Input: part model. Units: mm. Frame: model coordinates. A direction names the side the tool comes from. Round coordinates to 2 decimals unless told otherwise and drop trailing zeros. Order: outer loops, then holes, each group sorted by start corner. A loop starts at its lowest first (then second) coordinate and runs counter-clockwise, first axis right, second up.
Item 1: Cut plane D-D on y = -0.5. Output: boundary loops of the cut face in (x, z).
Item 2: Reachability of faces 1 (the flat face through (0, -33, 0)), 2 (the cylindrical face through (32.809, -3.2, 45.205)), 3 (the flat face through (-26.212, -3, 173)) from +Z, -Z, +X, -X, +Y, -Y: full face, straight path, thin tool, end or side. Return the list, or none.
Item 3: Line query: L1, parallel to X at y = 9, z = 141; L2, parallel to Y at x = 11.5, z = 141. Output: solid intervals per line, ascending.
Item 4: Cut plane C-C on z = 114.5. Output: boundary loops of the cut face in (x, y).
Item 5: Mould query, pull axis Y, two halves, no side actions, for faces 4 (the flat face through (-29.212, -3, 173)), 5 (the flat face through (2, -34.267, 173)), 6 (the flat face through (2, 29.233, 173)), 7 (the flat face through (2, 26.233, 173)). Classes: released by +Y, released by -Y, zero draft, split by the parting line, or undercut.
Item 6: Cut plane A-A on x = -7. Output: boundary loops of the cut face in (y, z), then the cut area to 3 significant figures.
Item 7: Cut plane B-B on y = 15.5. Output: boundary loops of the cut face in (x, z).
```python
from build123d import *

# Parameters (mm, degrees)
F0_W     = 63.5
F0_H     = 63.5
F0_W_2   = 57.5
F0_H_2   = 57.5
F1_DEPTH = 350
F2_R     = 5.25
F3_DEPTH = 10


with BuildPart() as f1:
    # F0 (on Top) → F1 (new body)
    with BuildSketch(Plane.XY):
        with Locations((2.538389, -2.516717)):
            Rectangle(F0_W, F0_H)
        with Locations((2.538389, -2.516717)):
            Rectangle(F0_W_2, F0_H_2, mode=Mode.SUBTRACT)
    extrude(amount=F1_DEPTH)

    # F2 (on face) → F3 (cut)
    with BuildSketch(Plane.YZ.offset(34.288389)):
        with Locations((-2.516717, 40)):
            Circle(F2_R)
    extrude(amount=-F3_DEPTH, mode=Mode.SUBTRACT)


solid = f1.part
```
From the geometry:
1. outline: (-29.21, 0) - (-26.21, 0) - (-26.21, 350) - (-29.21, 350) - close; (31.29, 0) - (34.29, 0) - (34.29, 35.15) - (31.29, 35.15) - close; (31.29, 44.85) - (34.29, 44.85) - (34.29, 350) - (31.29, 350) - close
2. face 1: -Z, +X, -X, +Y, -Y
2. face 2: +X
2. face 3: +Z, -Z
3. L1: x = -29.21 to -26.21, 31.29 to 34.29
3. L2: y = -34.27 to -31.27, 26.23 to 29.23
4. outline: (-29.21, -34.27) - (34.29, -34.27) - (34.29, 29.23) - (-29.21, 29.23) - close; hole (-26.21, -31.27) - (31.29, -31.27) - (31.29, 26.23) - (-26.21, 26.23) - close
5. face 4: zero draft
5. face 5: released by -Y
5. face 6: released by +Y
5. face 7: undercut
6. outline: (-34.27, 0) - (-31.27, 0) - (-31.27, 350) - (-34.27, 350) - close; (26.23, 0) - (29.23, 0) - (29.23, 350) - (26.23, 350) - close
6. area: 2,100 mm2
7. outline: (-29.21, 0) - (-26.21, 0) - (-26.21, 350) - (-29.21, 350) - close; (31.29, 0) - (34.29, 0) - (34.29, 350) - (31.29, 350) - close
